Geometry check sheet. Reference: the model listing, model coordinates, mm. Round coordinates to 2 decimals unless told otherwise and drop trailing zeros. Write each loop counter-clockwise with the first axis right and the second up, starting at its lowest first coordinate (ties: lowest second). Pieces come first, ordered by that corner, then holes. Notation, with made-up numbers: M -23,-9.75 L 10,-9.75 A23 cw 10,15.25 Z; hole C 58,7.5 d1. An arc over 180 degrees is marked long. One line per item, written item: value. Start each with the question number.
1. Section check B-B (x = 12.5). Record the boundary of the cut face in (y, z), and give its area (3 significant figures).
2. Section check C-C (y = -1.5). Record the boundary of the cut face in (x, z).
3. Section check D-D (y = -8). Count the separate pieces of the cut face and the enclosed holes in it, and give its area (3 significant figures).
4. Depth check by flat-ended pin: P1, Ø6.5, axis at y = -9, z = 2.5, coming from the -X side; P2, Ø4, axis at y = -8, z = 5, coming from the -X side; P3, Ø2, axis at y = -8, z = 5, coming from the -X side. Enter the tip coordinate at first touch or a pass-through.
5. Scan lines: probe 1 along Z at (x, y) = (35.9, -8); probe 2 along X at (y, z) = (-9.5, 6.5); probe 3 along Y at (x, z) = (13, 40.5). Record each from-to range of solid material in increasing order. Write a range as [from, to].
6. Section check A-A (z = 37.5). Record the boundary of the cut face in (x, y).
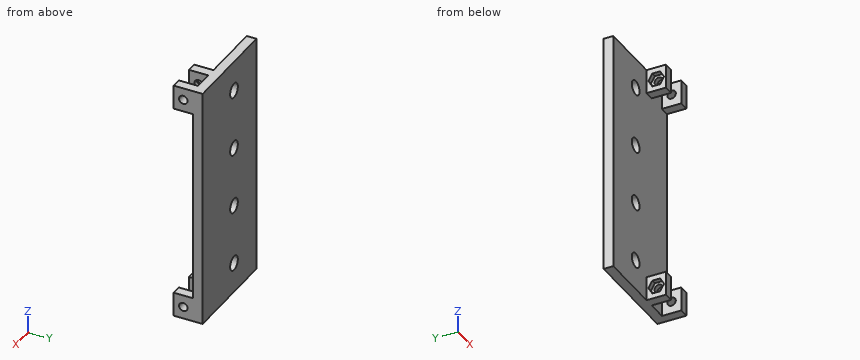
from build123d import *

# Parameters (mm, degrees)
F0_W      = 25
F0_H      = 100
F1_DEPTH  = 4
F2_W      = 4
F2_H      = 10
F3_DEPTH  = 8
F5_DEPTH  = 5
F4_R      = 3
F6_DEPTH  = 25
F8_DEPTH  = 12
F9_W      = 4
F9_H      = 100
F10_DEPTH = 8
F11_W     = 8
F11_H     = 80
F12_DEPTH = 25
F13_R     = 1.75
F14_DEPTH = 2
F15_DEPTH = 25


with BuildPart() as f1:
    # F0 (on Front) → F1 (new body)
    with BuildSketch(Plane.XZ):
        with Locations((12.5, 50)):
            Rectangle(F0_W, F0_H)
    extrude(amount=F1_DEPTH)

    # F2 (on face) → F3 (join)
    with BuildSketch(Plane.XZ.offset(4)):
        with Locations((23, 95)):
            Rectangle(F2_W, F2_H)
        with Locations((23, 5)):
            Rectangle(F2_W, F2_H)
    extrude(amount=F3_DEPTH)

    # F5 (add): a face of the model
    f5_faces = [f1.faces().sort_by_distance(p)[0] for p in [
        (0, -2, 50),
    ]]
    extrude(f5_faces, amount=F5_DEPTH)

    # F4 (on face) → F6 (cut)
    with BuildSketch(Plane(origin=(0, 0, 0), x_dir=(-1, 0, 0), z_dir=(0, 1, 0))):
        with Locations((-12.5, 12.5)):
            Circle(F4_R)
        with Locations((-12.5, 37.5)):
            Circle(F4_R)
        with Locations((-12.5, 62.5)):
            Circle(F4_R)
        with Locations((-12.5, 87.5)):
            Circle(F4_R)
    extrude(amount=-F6_DEPTH, mode=Mode.SUBTRACT)

    # F7 (on face) → F8 (join)
    with BuildSketch(Plane.YZ.offset(25)):
        Polygon((-4, 0), (0, 0), (0, 100), (-4, 100), (-4, 90), (-4, 10), align=None)
    extrude(amount=F8_DEPTH)

    # F9 (on face) → F10 (join, through all)
    with BuildSketch(Plane.XZ.offset(4)):
        with Locations((35, 50)):
            Rectangle(F9_W, F9_H)
    extrude(amount=F10_DEPTH)

    # F11 (on face) → F12 (cut)
    with BuildSketch(Plane(origin=(33, 0, 0), x_dir=(0, -1, 0), z_dir=(-1, 0, 0))):
        with Locations((8, 50)):
            Rectangle(F11_W, F11_H)
    extrude(amount=-F12_DEPTH, mode=Mode.SUBTRACT)

    # F13 (on face) → F14 (cut)
    with BuildSketch(Plane(origin=(21, 0, 0), x_dir=(0, -1, 0), z_dir=(-1, 0, 0))):
        Polygon((11.2331615075, 5), (9.6165807537, 7.8), (6.3834192463, 7.8), (4.7668384925, 5), (6.3834192463, 2.2), (9.6165807537, 2.2), align=None)
        with Locations((8, 5)):
            Circle(F13_R, mode=Mode.SUBTRACT)
        Polygon((9.6165807537, 92.2), (11.2331615075, 95), (9.6165807537, 97.8), (6.3834192463, 97.8), (4.7668384925, 95), (6.3834192463, 92.2), align=None)
        with Locations((8, 95)):
            Circle(F13_R, mode=Mode.SUBTRACT)
    extrude(amount=-F14_DEPTH, mode=Mode.SUBTRACT)

    # F13 (on face) → F15 (cut)
    with BuildSketch(Plane(origin=(21, 0, 0), x_dir=(0, -1, 0), z_dir=(-1, 0, 0))):
        with Locations((8, 5)):
            Circle(F13_R)
        with Locations((8, 95)):
            Circle(F13_R)
    extrude(amount=-F15_DEPTH, mode=Mode.SUBTRACT)


solid = f1.part
Result sheet:
1. outline: M -4,0 L 0,0 L 0,9.5 L -4,9.5 Z; M -4,15.5 L 0,15.5 L 0,34.5 L -4,34.5 Z; M -4,40.5 L 0,40.5 L 0,59.5 L -4,59.5 Z; M -4,65.5 L 0,65.5 L 0,84.5 L -4,84.5 Z; M -4,90.5 L 0,90.5 L 0,100 L -4,100 Z
1. area: 304 mm2
2. outline: M -5,0 L 37,0 L 37,100 L -5,100 Z; hole C 12.5,12.5 d6; hole C 12.5,37.5 d6; hole C 12.5,62.5 d6; hole C 12.5,87.5 d6
3. separate pieces: 8
3. enclosed holes: 0
3. area: 95.6 mm2
4. P1: stops at x = 21
4. P2: stops at x = 23
4. P3: passes through
5. probe 1: z = [0, 3.25], [6.75, 10], [90, 93.25], [96.75, 100]
5. probe 2: x = [23, 25], [33, 37]
5. probe 3: y = [-4, 0]
6. outline: M -5,-4 L 9.5,-4 L 9.5,0 L -5,0 Z; M 15.5,-4 L 37,-4 L 37,0 L 15.5,0 Z
